Input: part model. Units: mm. Frame: model coordinates. A direction names the side the tool comes from. Coordinates: 2 decimals unless noted, no trailing zeros. Order: outer loops, then holes, each group sorted by start corner. A loop starts at its lowest first (then second) coordinate and runs counter-clockwise, first axis right, second up. Notation, with made-up numbers: (-25, 0.5) -> (16, 0.5) arc R6 cw to (16, 9.5) -> close; hole circle Ø7 at (52, 60.25). An arc over 180 degrees is marked (long way). Use CSV: the item, a comma, the result in double quotes. Start each with the question number.
```python
from build123d import *
from build123d.topology import SkipClean

# Parameters (mm, degrees)
CROQUIS1_R              = 8.25
SALIENTE_EXTRUIR1_DEPTH = 5
CROQUIS2_R              = 4
SALIENTE_EXTRUIR2_DEPTH = 15


with BuildPart() as part:
    # Croquis1 → Saliente-Extruir1 (new body)
    with BuildSketch(Plane(origin=(0, 0, 0), x_dir=(1, 0, 0), z_dir=(0, 1, 0))):
        with Locations(Location((0, 0, 0), (0, 0, 270))):
            Circle(CROQUIS1_R)
        with BuildLine():
            Line((-2.6, 1.95), (2.6, 1.95))
            ThreePointArc((2.6, 1.95), (0, -3.25), (-2.6, 1.95))
        make_face(mode=Mode.SUBTRACT)
    extrude(amount=SALIENTE_EXTRUIR1_DEPTH)

    # Croquis2 → Saliente-Extruir2 (add)
    with SkipClean():  # the faces are left unmerged after this step: merging them gives an invalid solid
        with BuildSketch(Plane(origin=(0, 5, 0), x_dir=(1, 0, 0), z_dir=(0, 1, 0))):
            with Locations(Location((0, 0, 0), (0, 0, 270))):
                Circle(CROQUIS2_R)
            with BuildLine():
                Line((2.6, 1.95), (-2.6, 1.95))
                ThreePointArc((-2.6, 1.95), (0, -3.25), (2.6, 1.95))
            make_face(mode=Mode.SUBTRACT)
        extrude(amount=SALIENTE_EXTRUIR2_DEPTH)


solid = part.part
```
1. Section B-B on z = -0.5. Return loops of the section in (x, y), then the cut area to 3 significant figures.
2. Section C-C on y = 18.25. Return loops of the section in (x, z), then the cut area to 3 significant figures.
3. Contact query for flat-ended pins moving along their axis: P1, Ø4, axis at x = 2.5, y = 5.5, coming from the +Z side; P2, Ø3, axis at y = 11.5, z = -3, coming from the +X side; P3, Ø8, axis at x = -5.5, y = 9.5, coming from the +Z side; P4, Ø1.5, axis at y = 11.5, z = 5.5, coming from the -X side. Output: stop coordinate, or through.
4. Section A-A on x = 0. Return loops of the section in (y, z).
5. Material intervals for line 1 along X through (y, z) = (14.75, 0); line 2 along X through (y, z) = (1.25, 0); line 3 along Y through (x, z) = (7.5, -2.75), sorted ascending.
6. Access query for faces 1 (the face through (0, 20, -2.1)), 2 (the face through (-3.905, 12.395, -0.867)). Directions: +Z, -Z, +X, -X, +Y, -Y. A direction counts if a zero-diameter tool reaches every point of the face in a straight line with its end or side. Return the directions, or none.
7. Section D-D on z = -3.75. Return loops of the section in (x, y).
Values follow:
1,outline,"(-8.23, 0) -> (-3.21, 0) -> (-3.21, 20) -> (-3.97, 20) -> (-3.97, 5) -> (-8.23, 5) -> close; (3.21, 0) -> (8.23, 0) -> (8.23, 5) -> (3.97, 5) -> (3.97, 20) -> (3.21, 20) -> close"
1,area,"73.0 mm2"
2,outline,"circle Ø8 at (0, 0); hole (-2.6, -1.95) -> (2.6, -1.95) arc R3.25 ccw (long way) to start"
2,area,"21.8 mm2"
3,P1,"stops at z = 8.23"
3,P2,"stops at x = 3.71"
3,P3,"stops at z = 3.71"
3,P4,"passes through"
4,outline,"(0, -8.25) -> (5, -8.25) -> (5, -4) -> (20, -4) -> (20, -1.95) -> (0, -1.95) -> close; (0, 3.25) -> (20, 3.25) -> (20, 4) -> (5, 4) -> (5, 8.25) -> (0, 8.25) -> close"
5,line 1,"x = -4 to -3.25, 3.25 to 4"
5,line 2,"x = -8.25 to -3.25, 3.25 to 8.25"
5,line 3,"y = 0 to 5"
6,face 1,"+Z, -Z, +X, -X, +Y"
6,face 2,"+Y"
7,outline,"(-7.35, 0) -> (7.35, 0) -> (7.35, 5) -> (1.39, 5) -> (1.39, 20) -> (-1.39, 20) -> (-1.39, 5) -> (-7.35, 5) -> close"
